For this review, take the finished solid that the model builds, in its own axes (mm). A direction names the side the tool comes from. Give positions to 0.01 mm unless a question says otherwise; leave off trailing zeros. Write each loop counter-clockwise with the first axis right and the second up, starting at its lowest first coordinate (ties: lowest second). Pieces come first, ordered by that corner, then holes. Notation, with made-up numbers: M 89,86 L 148,86 A25 cw 148,118 Z; hole C 74.25,-11.75 d9. An arc over 180 degrees is marked long. One line per item, written item: value. Start each with the question number.
Item 1: Tool access review of faces 4 (the face through (-70.95, -1.1, 2.66)), 5 (the face through (284.915, -0.42, 2.662)): name each direction out of +Z, -Z, +X, -X, +Y, -Y from which nothing blocks a thin tool from reaching the whole face with its end or side.
Item 2: Consider section B-B, the plane z = 2. Give the number of separate pieces and of enclosed holes in the cut face, and give its area (3 significant figures).
Item 3: Consider section A-A, the plane x = 46. Write out the cut boundary in (y, z).
Item 4: Clearance check with flat-ended pins moving along their axes: pin 1 Ø1.5 at (y, z) = (0, 2) entering from +X; pin 2 Ø3.5 at (x, y) = (-37.13, 6.7) entering from -Z; pin 3 Ø8 at (x, y) = (-3.5, -27.5) entering from -Z; pin 4 Ø1.6 at (y, z) = (-42, 1.5) entering from -X. State where each tip first meets the part, or that it passes through.
Item 5: To check wall thickness, follow probe 1 along Y at (x, z) = (304, 4); probe 2 along Y at (x, z) = (208.5, 2.75); probe 3 along Y at (x, z) = (111, 4.45). State the ranges of each line that lie inside material, in increasing order.
Item 6: Mouldability with a two-part tool opening along Y and no side actions: class faces 1 (the face through (479.025, 1.099, 2.662)), 2 (the face through (208, -22, 0)), 3 (the face through (123.16, 0.42, 2.66)) as released by +Y, released by -Y, zero draft, split by the parting line, or undercut.
```python
from build123d import *

# Parameters (mm, degrees)
SKETCH3_R           = 7.5
SKETCH3_R_2         = 2.75
BOSS_EXTRUDE1_DEPTH = 5.4
SKETCH4_W           = 30
SKETCH4_H           = 5.4
CUT_EXTRUDE1_DEPTH  = 6.4


with BuildPart() as part:
    # Sketch3 → Boss-Extrude1 (new body)
    with BuildSketch(Plane.XY):
        with BuildLine():
            Line((-20.962749028, 50), (429.037250972, 50))
            ThreePointArc((429.037250972, 50), (479.037250972, 0), (429.037250972, -50))
            Line((429.037250972, -50), (-20.962749028, -50))
            ThreePointArc((-20.962749028, -50), (-70.962749028, 0), (-20.962749028, 50))
        make_face()
        with Locations((-20.962749028, 0)):
            Circle(SKETCH3_R, mode=Mode.SUBTRACT)
        with Locations((429.037250972, 0)):
            Circle(SKETCH3_R, mode=Mode.SUBTRACT)
        with Locations((-4.794857209, 6.696960066)):
            Circle(SKETCH3_R_2, mode=Mode.SUBTRACT)
        with Locations((-4.794857209, -6.696960066)):
            Circle(SKETCH3_R_2, mode=Mode.SUBTRACT)
        with Locations((-14.265788962, -16.167891819)):
            Circle(SKETCH3_R_2, mode=Mode.SUBTRACT)
        with Locations((-27.659709094, -16.167891819)):
            Circle(SKETCH3_R_2, mode=Mode.SUBTRACT)
        with Locations((-37.130640847, -6.696960066)):
            Circle(SKETCH3_R_2, mode=Mode.SUBTRACT)
        with Locations((-37.130640847, 6.696960066)):
            Circle(SKETCH3_R_2, mode=Mode.SUBTRACT)
        with Locations((-27.659709094, 16.167891819)):
            Circle(SKETCH3_R_2, mode=Mode.SUBTRACT)
        with Locations((-14.265788962, 16.167891819)):
            Circle(SKETCH3_R_2, mode=Mode.SUBTRACT)
        with Locations((455.037250972, 10)):
            Circle(SKETCH3_R_2, mode=Mode.SUBTRACT)
        with Locations((441.037250972, 24)):
            Circle(SKETCH3_R_2, mode=Mode.SUBTRACT)
        with Locations((421.037250972, 24)):
            Circle(SKETCH3_R_2, mode=Mode.SUBTRACT)
        with Locations((455.037250972, -10)):
            Circle(SKETCH3_R_2, mode=Mode.SUBTRACT)
        with Locations((441.037250972, -24)):
            Circle(SKETCH3_R_2, mode=Mode.SUBTRACT)
        with Locations((421.037250972, -24)):
            Circle(SKETCH3_R_2, mode=Mode.SUBTRACT)
        with BuildLine():
            Line((179.037250972, 19.094555463), (229.037250972, 19.094555463))
            ThreePointArc((229.037250972, 19.094555463), (248.131806435, 0), (229.037250972, -19.094555463))
            Line((229.037250972, -19.094555463), (179.037250972, -19.094555463))
            ThreePointArc((179.037250972, -19.094555463), (159.942695509, 0), (179.037250972, 19.094555463))
        make_face(mode=Mode.SUBTRACT)
        with BuildLine():
            Line((304.005250972, 19.094555463), (354.005250972, 19.094555463))
            ThreePointArc((354.005250972, 19.094555463), (373.099806435, 0), (354.005250972, -19.094555463))
            Line((354.005250972, -19.094555463), (304.005250972, -19.094555463))
            ThreePointArc((304.005250972, -19.094555463), (284.910695509, 0), (304.005250972, 19.094555463))
        make_face(mode=Mode.SUBTRACT)
        with BuildLine():
            Line((54.069250972, 19.094555463), (104.069250972, 19.094555463))
            ThreePointArc((104.069250972, 19.094555463), (123.163806435, 0), (104.069250972, -19.094555463))
            Line((104.069250972, -19.094555463), (54.069250972, -19.094555463))
            ThreePointArc((54.069250972, -19.094555463), (34.974695509, 0), (54.069250972, 19.094555463))
        make_face(mode=Mode.SUBTRACT)
    extrude(amount=BOSS_EXTRUDE1_DEPTH)

    # Sketch4 → Cut-Extrude1 (cut, through all)
    with BuildSketch(Plane.XY.offset(5.4)):
        with Locations((-5.962749028, 42.3)):
            Rectangle(SKETCH4_W, SKETCH4_H)
        with Locations((54.037250972, 42.3)):
            Rectangle(SKETCH4_W, SKETCH4_H)
        with Locations((114.037250972, 42.3)):
            Rectangle(SKETCH4_W, SKETCH4_H)
        with Locations((174.037250972, 42.3)):
            Rectangle(SKETCH4_W, SKETCH4_H)
        with Locations((234.037250972, 42.3)):
            Rectangle(SKETCH4_W, SKETCH4_H)
        with Locations((294.037250972, 42.3)):
            Rectangle(SKETCH4_W, SKETCH4_H)
        with Locations((354.037250972, 42.3)):
            Rectangle(SKETCH4_W, SKETCH4_H)
        with Locations((414.037250972, 42.3)):
            Rectangle(SKETCH4_W, SKETCH4_H)
        with Locations((414.037250972, -42.3)):
            Rectangle(SKETCH4_W, SKETCH4_H)
        with Locations((354.037250972, -42.3)):
            Rectangle(SKETCH4_W, SKETCH4_H)
        with Locations((294.037250972, -42.3)):
            Rectangle(SKETCH4_W, SKETCH4_H)
        with Locations((234.037250972, -42.3)):
            Rectangle(SKETCH4_W, SKETCH4_H)
        with Locations((174.037250972, -42.3)):
            Rectangle(SKETCH4_W, SKETCH4_H)
        with Locations((114.037250972, -42.3)):
            Rectangle(SKETCH4_W, SKETCH4_H)
        with Locations((54.037250972, -42.3)):
            Rectangle(SKETCH4_W, SKETCH4_H)
        with Locations((-5.962749028, -42.3)):
            Rectangle(SKETCH4_W, SKETCH4_H)
    extrude(amount=-CUT_EXTRUDE1_DEPTH, mode=Mode.SUBTRACT)


solid = part.part
```
Model answer:
1. face 4: +Z, -Z, -X
1. face 5: +Z, -Z
2. separate pieces: 1
2. enclosed holes: 35
2. area: 40,400 mm2
3. outline: M -50,0 L -45,0 L -45,5.4 L -50,5.4 Z; M -39.6,0 L -17.31,0 L -17.31,5.4 L -39.6,5.4 Z; M 17.31,0 L 39.6,0 L 39.6,5.4 L 17.31,5.4 Z; M 45,0 L 50,0 L 50,5.4 L 45,5.4 Z
4. pin 1: stops at x = 479.04
4. pin 2: passes through
4. pin 3: stops at z = 0
4. pin 4: stops at x = -49.29
5. probe 1: y = -50 to -45, -39.6 to -19.09, 19.09 to 39.6, 45 to 50
5. probe 2: y = -50 to -19.09, 19.09 to 50
5. probe 3: y = -50 to -45, -39.6 to -17.79, 17.79 to 39.6, 45 to 50
6. face 1: split by the parting line
6. face 2: zero draft
6. face 3: undercut
